Source: CAD feature listing. Evaluate the final solid. Frame: model axes, mm. Face numbers are marked on the shaded views. A direction names the side the tool comes from. Round coordinates to 2 decimals unless told otherwise and drop trailing zeros. Order: outer loops, then holes, each group sorted by start corner. A loop starts at its lowest first (then second) coordinate and runs counter-clockwise, first axis right, second up. Notation, with made-up numbers: (20.5, -0.5) -> (41.5, -0.5) arc R26 cw to (41.5, 14.5) -> close; hole circle Ø9 at (-26.75, 19). An arc over 180 degrees is marked (long way). Answer as CSV lines item,"result". Start each with the question number.
(1) Contact query for flat-ended pins moving along their axis: P1, Ø8, axis at x = -9, z = 45, coming from the -Y side; P2, Ø5.5, axis at x = -4.5, y = -85, coming from the -Z side; P3, Ø15, axis at x = 1, z = 81, coming from the +Y side; P4, Ø10, axis at x = 1, y = -84.5, coming from the +Z side. Output: stop coordinate, or through.
(2) Section query C-C (y = -125). Output: boundary loops of the cut face in (x, z), plus the area to 3 significant figures.
(3) Line query: line 1 along Z through (x, y) = (0, -92.1); line 2 along Y through (x, z) = (8.25, 72); line 3 along Y through (x, z) = (-8.5, -1) (3 decimals). Output: solid intervals per line, ascending. Write a range as from..to.
(4) Set-up query: the marked faces 4, 5, 6 and 7. Return all of +Z, -Z, +X, -X, +Y, -Y with unobstructed straight access to the full face (end or side cutting, diameter ignored); none if empty.
(5) Section query B-B (z = 53.5). Output: boundary loops of the cut face in (x, y) (1 decimal), plus the area to 3 significant figures.
(6) Section query A-A (y = -82.55). Output: boundary loops of the cut face in (x, z) (3 decimals).
(7) Pull-direction query (Z, two-part tool) for the marked faces 1, 2 and 3; classes: +Z half, -Z half, draft (parallel to the pull), parting line (faces both ways), or undercut.
```python
from build123d import *

# Parameters (mm, degrees)
F0_R      = 6.35
F1_DEPTH  = 152.4
F4_R      = 12.7
F5_DEPTH  = 6.35
F6_R      = 12.7
F7_DEPTH  = 6.35
F9_R      = 6.35
F10_DEPTH = 50.8
F11_W     = 19.05
F11_H     = 28.575
F12_DEPTH = 38.1
F13_W     = 12.7
F13_H     = 28.575
F14_DEPTH = 25.4
F15_R     = 4.7625
F16_DEPTH = 25.4


with BuildPart() as f1:
    # F0 (on Front) → F1 (new body)
    with BuildSketch(Plane.XZ):
        Circle(F0_R)
    extrude(amount=F1_DEPTH)

    # F4 (on offset) → F5 (join)
    with BuildSketch(Plane.XZ.offset(127)):
        Circle(F4_R)
    extrude(amount=F5_DEPTH)

    # F6 (on offset) → F7 (join)
    with BuildSketch(Plane.XZ.offset(34.925)):
        Circle(F6_R)
    extrude(amount=F7_DEPTH)

    # F9 (on offset) → F10 (join)
    with BuildSketch(Plane.XY):
        with Locations((0, -82.55)):
            Circle(F9_R)
    extrude(amount=F10_DEPTH)

    # F11 (on face) → F12 (join)
    with BuildSketch(Plane.XY.offset(50.8)):
        with Locations((0, -82.55)):
            Rectangle(F11_W, F11_H)
    extrude(amount=F12_DEPTH)

    # F13 (on face) → F14 (cut)
    with BuildSketch(Plane(origin=(-9.525, 0, 0), x_dir=(0, -1, 0), z_dir=(-1, 0, 0))):
        with Locations((82.55, 74.6125)):
            Rectangle(F13_W, F13_H)
    extrude(amount=-F14_DEPTH, mode=Mode.SUBTRACT)

    # F15 (on face) → F16 (cut)
    with BuildSketch(Plane(origin=(0, -68.2625, 0), x_dir=(-1, 0, 0), z_dir=(0, 1, 0))):
        with Locations((0, 79.375)):
            Circle(F15_R)
    extrude(amount=-F16_DEPTH, mode=Mode.SUBTRACT)


solid = f1.part
```
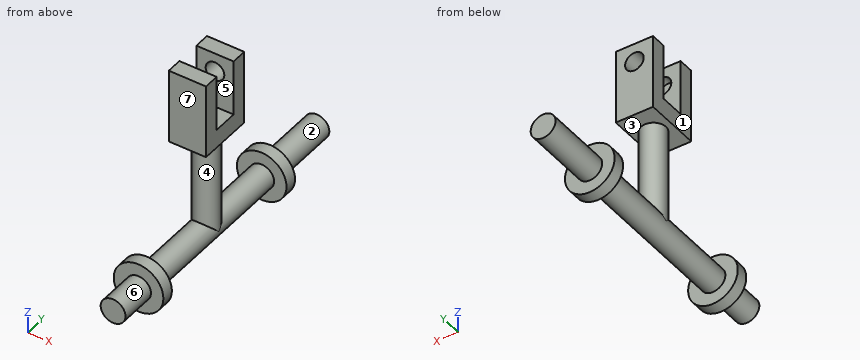
Answer block:
1,P1,"y = -86.46"
1,P2,"z = -6.1"
1,P3,"y = -68.26"
1,P4,"z = 88.9"
2,outline,"circle Ø12.7 at (0, 0)"
2,area,"127 mm2"
3,line 1,"-6.35..6.35, 50.8..74.61, 84.14..88.9"
3,line 2,"-96.84..-88.9, -76.2..-68.26"
3,line 3,"-133.35..-127, -41.275..-34.925"
4,face 4,"none"
4,face 5,"+Z, +X, -X"
4,face 6,"-Y"
4,face 7,"+Z, +X, -X, -Y"
5,outline,"(-9.5, -96.8) -> (9.5, -96.8) -> (9.5, -68.3) -> (-9.5, -68.3) -> close"
5,area,"544 mm2"
6,outline,"(-9.525, 50.8) -> (-6.35, 50.8) -> (-6.35, 0) arc R6.35 ccw to (6.35, 0) -> (6.35, 50.8) -> (9.525, 50.8) -> (9.525, 60.325) -> (-9.525, 60.325) -> close"
7,face 1,"draft"
7,face 2,"parting line"
7,face 3,"undercut"
